Answer from the drawing. Dimensions are ordinates in mm from the lowest x, y and z of the part. A direction names the side the tool comes from. Round coordinates to 2 decimals unless told otherwise and drop trailing zeros. Write each loop counter-clockwise with the first axis right and the second up, starting at its lowest first coordinate (ties: lowest second). Pieces come first, ordered by that corner, then holes. Notation, with made-up numbers: (-23, -5.5) -> (8, -5.5) arc R9 ccw to (8, 7.5) -> close; hole circle Ø9 at (33.25, -8.5). An arc over 180 degrees is marked (long way). Return JSON: item names as keys, results as strings. Group by question number.
(1) For the marked faces 1, 2, 3, 4 and 5, determine the directions among +Z, -Z, +X, -X, +Y, -Y from which every point of the face is accessible in a straight line to the end or side of a thin tool.
(2) The mould has two halves that part along Z. Classify the marked faces 6, 7 and 8: released by +Z, released by -Z, zero draft, split by the parting line, or undercut.
(3) Straight lines are drawn through the part: line 1 (Y direction, x = 1.05, z = 4.75); line 2 (Y direction, x = 1.75, z = 2.25). For each, find the intervals that lie inside material, in ascending order.
(4) Given pin 1 (0.9 mm diameter, centred on x = 1, z = 12, fed in from -Y); pin 2 (0.9 mm diameter, centred on x = 1, z = 1, fed in from -Y); pin 3 (1.5 mm diameter, centred on x = 2, y = 1, fed in from -Z), each flat-ended and moving along its own axis, determine where each tip first touches the part or whether it passes through.
(5) A cutting plane is placed at B-B on z = 12.5. Give the vertices of the cut face in (x, y).
(6) A cutting plane is placed at C-C on y = 8.75. Give the vertices of the cut face in (x, z).
(7) A cutting plane is placed at A-A on x = 1.8. Give the vertices of the cut face in (y, z) (1 decimal), then the cut area to 3 significant figures.
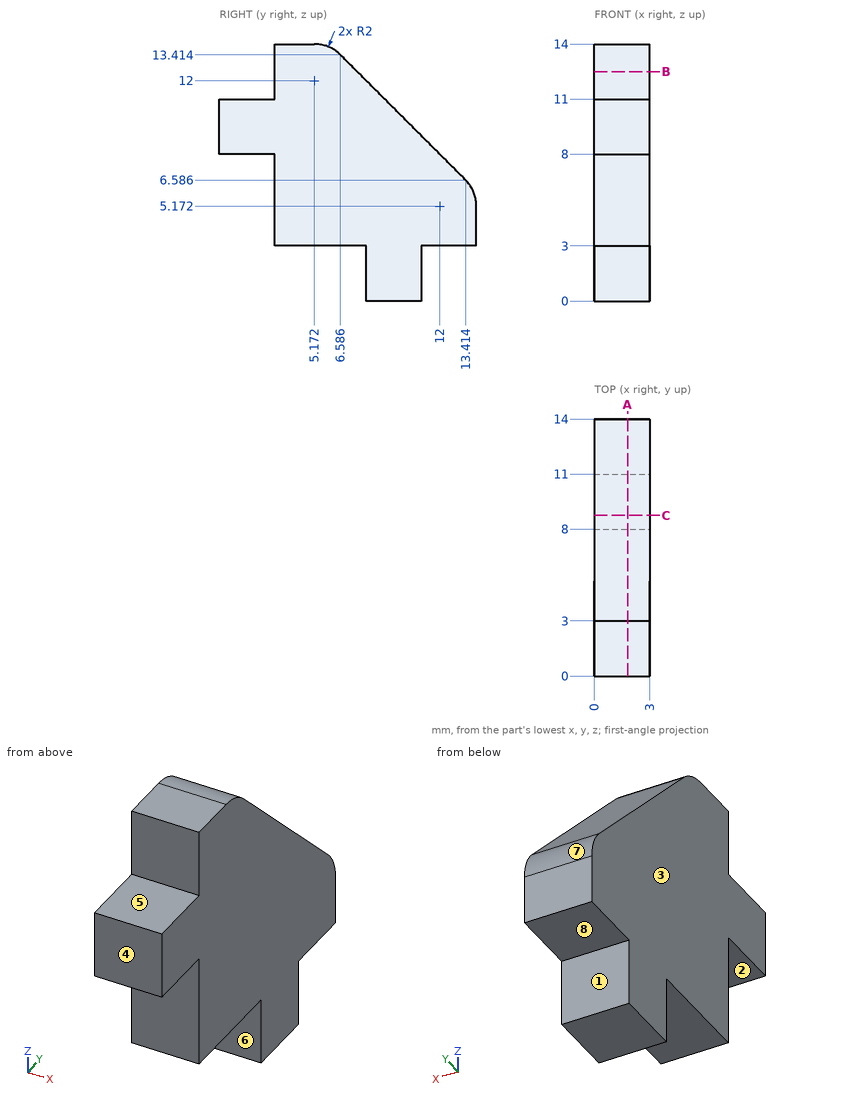
Checks:
{
 "1": {"face 1": "-Z, +X, -X, +Y", "face 2": "-Z, +X, -X, -Y", "face 3": "+Z, -Z, -X, +Y, -Y", "face 4": "+Z, -Z, +X, -X, -Y", "face 5": "+Z, +X, -X, -Y"},
 "2": {"face 6": "zero draft", "face 7": "released by +Z", "face 8": "released by -Z"},
 "3": {"line 1": "y = 3 to 14", "line 2": "y = 8 to 11"},
 "4": {"pin 1": "stops at y = 3", "pin 2": "stops at y = 8", "pin 3": "stops at z = 8"},
 "5": {"outline": "(0, 3) -> (3, 3) -> (3, 7.5) -> (0, 7.5) -> close"},
 "6": {"outline": "(0, 0) -> (3, 0) -> (3, 11.25) -> (0, 11.25) -> close"},
 "7": {"outline": "(0, 8) -> (3, 8) -> (3, 3) -> (8, 3) -> (8, 0) -> (11, 0) -> (11, 3) -> (14, 3) -> (14, 5.2) arc R2 ccw to (13.4, 6.6) -> (6.6, 13.4) arc R2 ccw to (5.2, 14) -> (3, 14) -> (3, 11) -> (0, 11) -> close", "area": "107 mm^2"}
}
